from build123d import *

# Parameters (mm, degrees)
SKETCH_W           = 3.81
SKETCH_H           = 3.81
SKETCH_W_2         = 3.2258
SKETCH_H_2         = 2.2098
PAD_DEPTH          = 2.54
SKETCH001_R        = 4.7625
PAD001_DEPTH       = 2.54
FILLET_R           = 0.254
FILLET_FACE14_W    = 2.2098
FILLET_FACE14_H    = 3.2258
POCKET_DEPTH       = 2.286
POCKET_FACE11_W    = 3.81
POCKET_FACE11_H    = 3.81
POCKET_FACE11_W_2  = 2.2098
POCKET_FACE11_H_2  = 3.2258
POCKET001_DEPTH    = 2.286
POCKET001_FACE11_R = 4.7625
POCKET001_FACE11_W = 3.81
POCKET001_FACE11_H = 3.81
PAD002_DEPTH       = 0.254


with BuildPart() as part:
    # Sketch → Pad (new body)
    with BuildSketch(Plane.XY):
        Rectangle(SKETCH_W, SKETCH_H)
        Rectangle(SKETCH_W_2, SKETCH_H_2, mode=Mode.SUBTRACT)
    extrude(amount=PAD_DEPTH)

    # Sketch001 (on Face10 of Pad) → Pad001 (join)
    with BuildSketch(Plane.XY.offset(2.54)):
        Circle(SKETCH001_R)
    extrude(amount=PAD001_DEPTH)

    # Fillet
    fillet_edges = [part.edges().sort_by_distance(p)[0] for p in [
        (-4.7625, 0, 5.08),
    ]]
    fillet(fillet_edges, radius=FILLET_R)

    # Fillet Face14 → Pocket (cut)
    with BuildSketch(Plane(origin=(0, 0, 2.54), x_dir=(0, -1, 0), z_dir=(0, 0, -1))):
        Rectangle(FILLET_FACE14_W, FILLET_FACE14_H)
    extrude(amount=-POCKET_DEPTH, mode=Mode.SUBTRACT)

    # Pocket Face11 → Pocket001 (cut)
    with BuildSketch(Plane(origin=(0, 0, 0), x_dir=(0, -1, 0), z_dir=(0, 0, -1))):
        Rectangle(POCKET_FACE11_W, POCKET_FACE11_H)
        Rectangle(POCKET_FACE11_W_2, POCKET_FACE11_H_2, mode=Mode.SUBTRACT)
    extrude(amount=-POCKET001_DEPTH, mode=Mode.SUBTRACT)

    # Pocket001 Face11 → Pad002 (add)
    with BuildSketch(Plane(origin=(0, 0, 2.54), x_dir=(0, -1, 0), z_dir=(0, 0, -1))):
        Circle(POCKET001_FACE11_R)
        Rectangle(POCKET001_FACE11_W, POCKET001_FACE11_H, mode=Mode.SUBTRACT)
    extrude(amount=PAD002_DEPTH)


solid = part.part
Read the model definition and answer for the solid it produces. Units are mm, in the model's axes. Round coordinates to 2 decimals unless told otherwise and drop trailing zeros. Loops run counter-clockwise (first coordinate to the right, second up) from the corner with the lowest first, then second, coordinate; pieces in that order, holes last.
Q1. Consider probe 1 along Y at (x, z) = (0, 2.75); probe 2 along Z at (x, y) = (-0.5, -0.5); probe 3 along X at (y, z) = (1, 3.95). Determine where each line is inside the solid, lowest interval first.
Q2. Section B-B on y = 0 is taken. Write down the section's boundary in (x, z), and give its area (3 significant figures).
Q3. Each of these flat-tipped pins is pushed along its axis until it touches: pin 1 (1 mm diameter, centred on y = -3.5, z = 3, fed in from -X); pin 2 (0.7 mm diameter, centred on y = -0.5, z = 3.5, fed in from +X). Where does it stop, or does it pass through?
Q4. Section A-A on z = 4.6 is taken. Write down the section's boundary in (x, y) (1 decimal), and give its area (3 significant figures).
Q5. Determine the mould class of faces 1 (the face through (1.613, 0, 4)), 2 (the face through (0, 1.105, 4)), 3 (the face through (0, 0, 5.08)) for opening direction X: released by +X, released by -X, zero draft, split by the parting line, or undercut.
Q6. Section C-C on x = 0 is taken. Write down the section's boundary in (y, z), and give its area (3 significant figures).
Output:
1. probe 1: y = -4.76 to -1.1, 1.1 to 4.76
1. probe 2: z = 4.83 to 5.08
1. probe 3: x = -4.66 to -1.61, 1.61 to 4.66
2. outline: (-4.76, 2.29) - (-1.61, 2.29) - (-1.61, 4.83) - (1.61, 4.83) - (1.61, 2.29) - (4.76, 2.29) - (4.76, 4.83) arc R0.25 ccw to (4.51, 5.08) - (-4.51, 5.08) arc R0.25 ccw to (-4.76, 4.83) - close
2. area: 18.4 mm2
3. pin 1: stops at x = -3.7
3. pin 2: stops at x = 4.76
4. outline: circle Ø9.5 at (0, 0); hole (-1.6, -1.1) - (1.6, -1.1) - (1.6, 1.1) - (-1.6, 1.1) - close
4. area: 64.1 mm2
5. face 1: undercut
5. face 2: undercut
5. face 3: zero draft
6. outline: (-4.76, 2.29) - (-1.1, 2.29) - (-1.1, 4.83) - (1.1, 4.83) - (1.1, 2.29) - (4.76, 2.29) - (4.76, 4.83) arc R0.25 ccw to (4.51, 5.08) - (-4.51, 5.08) arc R0.25 ccw to (-4.76, 4.83) - close
6. area: 21.0 mm2
